from build123d import *

# Parameters (mm, degrees)
FILLET1_R = 10
FILLET2_R = 1


with BuildPart() as part:
    # Sketch1 → Revolve1 (revolve)
    with BuildSketch(Plane(origin=(0, 0, 0), x_dir=(1, 0, 0), z_dir=(0, 1, 0))):
        with BuildLine():
            Line((4.350194802, 0.893), (3.17642875, 10.7482))
            Line((3.17642875, 10.7482), (3.748185925, 10.7482))
            Line((3.748185925, 10.7482), (3.748185925, 10.8752))
            Line((3.748185925, 10.8752), (3.17642875, 15.6758))
            Line((3.17642875, 15.6758), (3.748185925, 15.6758))
            Line((3.748185925, 15.6758), (3.748185925, 15.8028))
            Line((3.748185925, 15.8028), (3.17642875, 20.6034))
            Line((3.17642875, 20.6034), (3.748185925, 20.6034))
            Line((3.748185925, 20.6034), (3.748185925, 20.7304))
            Line((3.748185925, 20.7304), (3.189766531, 25.419013037))
            add(Edge.make_bspline(
                [(3.189766531, 25.419013037), (3.186366459, 25.447560793), (3.171391458, 25.478531163), (3.122909051, 25.520829006), (3.091096062, 25.531), (3.063600271, 25.531)],
                knots=[0, 0, 0, 0, 0.5, 0.5, 1, 1, 1, 1], degree=3))
            Line((3.063600271, 25.531), (2.248911555, 25.531))
            Line((2.248911555, 25.531), (2.248911555, -1.107))
            Line((2.248911555, -1.107), (5.5, -1.107))
            ThreePointArc((5.5, -1.107), (12.571067812, -4.035932188), (15.5, -11.107))
            Line((15.5, -11.107), (15.5, -29.102833044))
            Line((15.5, -29.102833044), (17.5, -29.102833044))
            Line((17.5, -29.102833044), (17.5, -11.107))
            ThreePointArc((17.5, -11.107), (13.985281374, -2.621718626), (5.5, 0.893))
            Line((5.5, 0.893), (4.350194802, 0.893))
        make_face()
    revolve(axis=Axis((0, 0, -25.781), (0, 0, 1)))

    # Fillet1
    fillet1_edges = [part.edges().sort_by_distance(p)[0] for p in [
        (-4.350194802, 0, -0.893),
    ]]
    fillet(fillet1_edges, radius=FILLET1_R)

    # Fillet2
    fillet2_edges = [part.edges().sort_by_distance(p)[0] for p in [
        (-2.248911555, 0, 1.107),
    ]]
    fillet(fillet2_edges, radius=FILLET2_R)


solid = part.part
Work out the finished part from the listing and answer in its coordinate system (mm). A direction names the side the tool comes from. Coordinates: 2 decimals unless noted, no trailing zeros. Write each loop counter-clockwise with the first axis right and the second up, starting at its lowest first coordinate (ties: lowest second). Pieces come first, ordered by that corner, then holes.
1. Flat-ended cylindrical pins translate along their axes: pin 1 (2 mm diameter, centred on x = 0.5, y = -1.5, fed in from +Z); pin 2 (4 mm diameter, centred on y = 6, z = 5, fed in from +X); pin 3 (8 mm diameter, centred on x = 0.5, y = -1.5, fed in from +Z). Find the tip coordinate at first contact, or state that the pin passes through.
Results list:
pin 1: stops at z = 0.85
pin 2: stops at x = 15.91
pin 3: stops at z = 1.11
2. The part is cut by section A-A, the plane z = -14. Write down the section's boundary in (x, y), and give its area (3 significant figures).
Results list:
outline: circle Ø6.75 at (0, 0); hole circle Ø4.5 at (0, 0)
area: 19.9 mm2
3. For faces 1 (the flat face through (-4, 0, 1.107)), 2 (the flat face through (7, -14, 29.103)), 3 (the conical face through (-0.442, 3.366, -13.843)), determine the directions among +Z, -Z, +X, -X, +Y, -Y from which every point of the face is accessible in a straight line to the end or side of a thin tool.
Results list:
face 1: +Z
face 2: +Z, +X, -X, +Y, -Y
face 3: none
4. For a pull along Y with two mould halves and no side action, classify faces 4 (the flat face through (-2, 2, -25.531)), 5 (the cylindrical face through (-13.887, -10.648, 19.979)), 6 (the cylindrical face through (-2.018, 15.368, 20.231)), 7 (the cylindrical face through (1.038, -1.995, -12.533)) as +Y half, -Y half, draft (parallel to the pull), parting line (faces both ways), or undercut.
Results list:
face 4: draft
face 5: parting line
face 6: undercut
face 7: undercut
5. Consider line 1 along Y through (x, z) = (0, 21.75); line 2 along Y through (x, z) = (0, -10); line 3 along X through (y, z) = (-3, 10). Determine where each line is inside the solid, lowest interval first.
Results list:
line 1: y = -17.5 to -15.5, 15.5 to 17.5
line 2: y = -3.27 to -2.25, 2.25 to 3.27
line 3: x = -17.19 to -15.14, 15.14 to 17.19
